from build123d import *

# Parameters (mm, degrees)
SKETCH1_R               = 1.5
BOSS_EXTRUDE1_DEPTH     = 1.5
SKETCH5_W               = 7.463090523
SKETCH5_H               = 8
BOSS_EXTRUDE2_DEPTH     = 3.5
CUT_EXTRUDE1_DEPTH      = 7
CUT_EXTRUDE1_DEPTH_BACK = 6
SKETCH2_W               = 2.5
SKETCH2_H               = 5.25
SKETCH3_R               = 2
CUT_EXTRUDE2_DEPTH      = 3
SKETCH6_W               = 5
SKETCH6_H               = 4
CUT_EXTRUDE3_DEPTH      = 3.5
SKETCH7_R               = 1.45
BOSS_EXTRUDE3_DEPTH     = 2.1


with BuildPart() as part:
    # Sketch1 → Boss-Extrude1 (new, symmetric)
    with BuildSketch(Plane.XY):
        with BuildLine():
            Line((12, 4), (0, 4))
            ThreePointArc((0, 4), (-4, 0), (0, -4))
            Line((0, -4), (12, -4))
            Line((12, -4), (12, 4))
        make_face()
        Circle(SKETCH1_R, mode=Mode.SUBTRACT)
    extrude(amount=BOSS_EXTRUDE1_DEPTH, both=True)

    # Sketch5 → Boss-Extrude2 (add, symmetric)
    with BuildSketch(Plane.XY):
        with Locations((8.268454739, 0)):
            Rectangle(SKETCH5_W, SKETCH5_H)
    extrude(amount=BOSS_EXTRUDE2_DEPTH, both=True)

    # Sketch2 → Cut-Extrude1 (cut, two sides: drawn at the far end of the back side and taken through both)
    with BuildSketch(Plane.XY.offset(1.5).offset(-CUT_EXTRUDE1_DEPTH_BACK)):
        with Locations((8.25, 0)):
            Rectangle(SKETCH2_W, SKETCH2_H)
    extrude(amount=CUT_EXTRUDE1_DEPTH + CUT_EXTRUDE1_DEPTH_BACK, mode=Mode.SUBTRACT)

    # Sketch3 → Cut-Extrude2 (cut)
    with BuildSketch(Plane(origin=(12, 0, 0), x_dir=(0, 0, -1), z_dir=(1, 0, 0))):
        with Locations(Location((0, 0, 0), (0, 0, 90))):
            Circle(SKETCH3_R)
    extrude(amount=-CUT_EXTRUDE2_DEPTH, mode=Mode.SUBTRACT)

    # Sketch6 → Cut-Extrude3 (cut)
    with BuildSketch(Plane(origin=(0, 0, -3.5), x_dir=(-1, 0, 0), z_dir=(0, 0, -1))):
        with Locations((-12, 0)):
            Rectangle(SKETCH6_W, SKETCH6_H)
    extrude(amount=-CUT_EXTRUDE3_DEPTH, mode=Mode.SUBTRACT)

    # Sketch7 → Boss-Extrude3 (add)
    with BuildSketch(Plane(origin=(0, 4, 0), x_dir=(1, 0, 0), z_dir=(0, 1, 0))):
        with Locations(Location((8.268454739, 0, 0), (0, 0, 180))):
            Circle(SKETCH7_R)
    extrude(amount=BOSS_EXTRUDE3_DEPTH)


solid = part.part
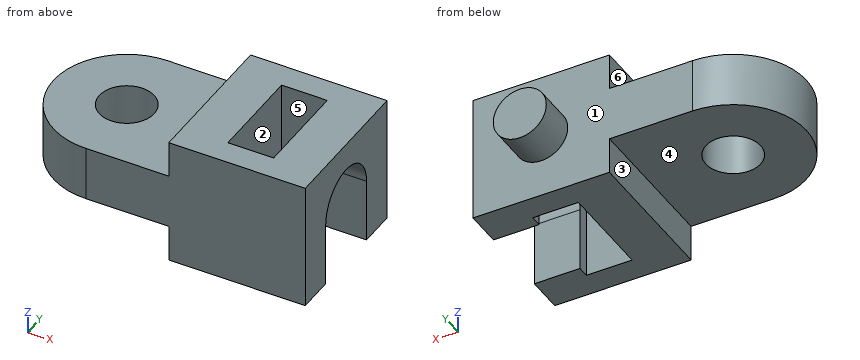
The listing builds one solid part. Answer for the finished solid, in the listing's coordinates (mm). Face numbers are marked on the shaded views. A direction names the side the tool comes from. Coordinates: 2 decimals unless noted, no trailing zeros. Loops run counter-clockwise (first coordinate to the right, second up) from the corner with the lowest first, then second, coordinate; pieces in that order, holes last. Notation, with made-up numbers: (88.5, 0.25) -> (106.5, 0.25) arc R16 cw to (106.5, 28.25) -> close; hole circle Ø11 at (42.25, 56). An arc over 180 degrees is marked (long way). Answer in a Markdown table with one row per item. Add a question column.
1. For the marked faces 4, 5 and 6, determine the directions among +Z, -Z, +X, -X, +Y, -Y from which every point of the face is accessible in a straight line to the end or side of a thin tool.
2. The part is cut by section D-D, the plane z = -2. Write down the section's boundary in (x, y) (3 decimals).
3. The part is cut by section B-B, the plane z = 2.25. Write down the section's boundary in (x, y) (3 decimals), then the cut area to 3 significant figures.
4. Flat-ended cylindrical pins translate along their axes: P1, Ø1, axis at x = 2, y = 3.5, coming from the +Z side; P2, Ø2.5, axis at x = 0, y = 0, coming from the -Z side; P3, Ø4, axis at y = -1.5, z = -1.5, coming from the +X side; P4, Ø4, axis at x = -0.5, y = 2, coming from the -Z side. Find the tip coordinate at first contact, or state that the pin passes through.
5. Determine the mould class of the marked faces 1, 2 and 3 for opening direction Y: +Y half, -Y half, draft (parallel to the pull), parting line (faces both ways), or undercut.
6. Consider line 1 (Y direction, x = 0, z = -0.7); line 2 (X direction, y = -2.25, z = -2.75); line 3 (Y direction, x = 1.75, z = 0). Determine where each line is inside the solid, lowest interval first. Write a range as [from, to].
7. The part is cut by section A-A, the plane y = 0. Write down the section's boundary in (x, z).
8. The part is cut by section C-C, the plane x = 8.5. Write down the section's boundary in (y, z) (3 decimals), then the cut area to 3 significant figures.
Answer below:
| question | item | result |
|---|---|---|
| 1 | face 4 | -Z, -X, +Y, -Y |
| 1 | face 5 | +Z, -Z |
| 1 | face 6 | +Z, -X, +Y, -Y |
| 2 | outline | (4.537, -4) -> (12, -4) -> (12, -2) -> (9.5, -2) -> (9.5, -2.625) -> (7, -2.625) -> (7, 2.625) -> (9.5, 2.625) -> (9.5, 2) -> (12, 2) -> (12, 4) -> (4.537, 4) -> close |
| 3 | outline | (4.537, -4) -> (12, -4) -> (12, 4) -> (4.537, 4) -> close; hole (7, -2.625) -> (9.5, -2.625) -> (9.5, 2.625) -> (7, 2.625) -> close |
| 3 | area | 46.6 mm2 |
| 4 | P1 | z = 1.5 |
| 4 | P2 | through |
| 4 | P3 | x = 12 |
| 4 | P4 | z = -1.5 |
| 5 | face 1 | +Y half |
| 5 | face 2 | undercut |
| 5 | face 3 | draft |
| 6 | line 1 | [-4, -1.5], [1.5, 4] |
| 6 | line 2 | [4.54, 7], [9.5, 12] |
| 6 | line 3 | [-4, 4] |
| 7 | outline | (-4, -1.5) -> (-1.5, -1.5) -> (-1.5, 1.5) -> (-4, 1.5) -> close; (1.5, -1.5) -> (4.54, -1.5) -> (4.54, -3.5) -> (7, -3.5) -> (7, 3.5) -> (4.54, 3.5) -> (4.54, 1.5) -> (1.5, 1.5) -> close; (9.5, 2) -> (12, 2) -> (12, 3.5) -> (9.5, 3.5) -> close |
| 8 | outline | (-4, -3.5) -> (-2.625, -3.5) -> (-2.625, 3.5) -> (-4, 3.5) -> close; (2.625, -3.5) -> (4, -3.5) -> (4, -1.431) -> (6.1, -1.431) -> (6.1, 1.431) -> (4, 1.431) -> (4, 3.5) -> (2.625, 3.5) -> close |
| 8 | area | 25.3 mm2 |
